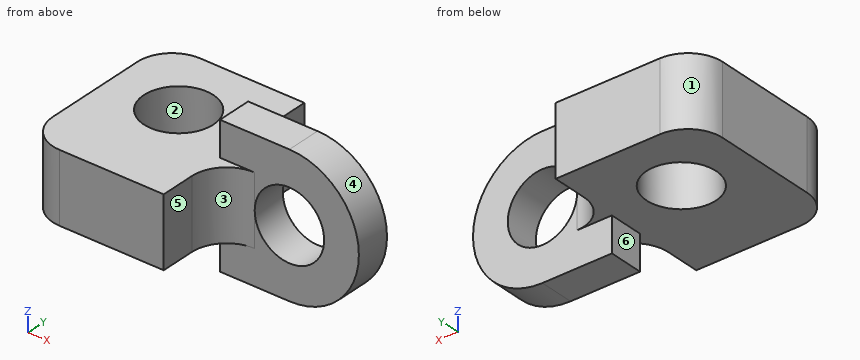
Autodesk Inventor part; units mm, degrees
ref_plane "工作平面1" through (0, 0, -10) normal (0, -1, 0) x (1, 0, 0)
ref_plane "YZ Plane" through (0, 0, 0) normal (1, 0, 0) x (0, 1, 0)
ref_plane "XZ Plane" through (0, 0, 0) normal (0, 1, 0) x (-1, 0, 0)
sketch "草圖1" plane through (0, 0, 0) normal (0, 0, 1) x (1, 0, 0)
  line L0 (-40, 25) -> (0, 25)
  line L1 (0, 25) -> (0, -25)
  line L2 (0, -25) -> (-40, -25)
  line L3 (-40, -25) -> (-40, 25)
  point P0 (0, 0)
  point P1 (0, 0)
  dimension "d0" = 50
  dimension "d1" = 40
extrude "擠出1" add sketch "草圖1" along normal mid plane 20
fillet "圓角1" radius 10 2 edges at (-40, 25, 0) (-40, -25, 0)
sketch "草圖2" plane through (0, 0, 10) normal (0, 0, 1) x (1, 0, 0)
  arc A0 (-40, -15) -> (-30, -25) centre (-30, -15) ccw
  line L0 (-40, -15) -> (-40, 15)
  arc A1 (-30, 25) -> (-40, 15) centre (-30, 15) ccw
  line L1 (-30, 25) -> (0, 25)
  line L2 (0, 25) -> (0, -25)
  line L3 (0, -25) -> (-30, -25)
  point P0 (0, 0)
  point P1 (-20, 5)
  dimension "d5" = 20
  dimension "d6" = 20
hole "孔1" at (-20, 5, 10) direction (0, 0, -1) diameter 20 end through all
ref_plane "工作平面1" through (0, 0, -10) normal (0, -1, 0) x (1, 0, 0)
sketch "草圖3" plane through (0, 0, -10) normal (0, -1, 0) x (1, 0, 0)
  line L0 (-11.3397, 0) -> (-11.3397, 20)
  line L1 (-11.3397, 20) -> (0, 20)
  line L2 (0, 20) -> (0, 0)
  line L3 (0, 0) -> (-11.3397, 0)
  line L4 (-28.6603, 20) -> (-28.6603, 0)
  line L5 (-28.6603, 0) -> (-40, 0)
  line L6 (-40, 0) -> (-40, 20)
  line L7 (-40, 20) -> (-28.6603, 20)
  circle A0 centre (20, 10) radius 20
  line L8 (20, -10) -> (0, -10)
  line L9 (0, -10) -> (0, 30)
  line L10 (0, 30) -> (20, 30)
  line L11 (20, 30) -> (20, -10)
  point P0 (0, 10)
  point P1 (0, 10)
  point P2 (20, 10)
  point P3 (0, 20)
  dimension "d15" = 40
  dimension "d14" = 20
extrude "擠出2" add sketch "草圖3" along normal mid plane 10 contours L2 A0 L8 L9 | L9 L10 A0 L2 | A0 L11 | A0 L11
fillet "圓角2" radius 10 2 edges at (0, 5, 0) (0, -5, 0)
sketch "草圖4" plane through (0, 5, -10) normal (0, 1, 0) x (1, 0, 0)
  arc A0 (20, -30) -> (20, 10) centre (20, -10) ccw
  point P0 (0, -10)
hole "孔2" at (20, 5, 0) direction (0, -1, 0) diameter 20 end through all
properties part number "22" material "鋼、碳鋼"
Read the model definition and answer for the solid it produces. Units are mm, in the model's axes. Face numbers are marked on the shaded views. A direction names the side the tool comes from. Give positions to 0.01 mm unless a question says otherwise; leave off trailing zeros. Loops run counter-clockwise (first coordinate to the right, second up) from the corner with the lowest first, then second, coordinate; pieces in that order, holes last. Notation, with made-up numbers: M 55.25,46 L 97.25,46 A17 ccw 97.25,60 Z; hole C -33,51.5 d9. An arc over 180 degrees is marked long. Write each question's results on one line, items separated by ' | '.
1. Section C-C on z = 1 is taken. Give the vertices of the cut face in (x, y), plus the area to 3 significant figures.
Values:
outline: M -40,-15 A10 ccw -30,-25 L 0,-25 L 0,-15 A10 cw 10,-5 L 10.05,-5 L 10.05,5 L 10,5 A10 cw 0,15 L 0,25 L -30,25 A10 ccw -40,15 Z; M 29.95,-5 L 39.97,-5 L 39.97,5 L 29.95,5 Z; hole C -20,5 d20 | area: 1,890 mm^2
2. Section D-D on y = 20 is taken. Give the vertices of the cut face in (x, z).
Values:
outline: M -38.66,-10 L 0,-10 L 0,10 L -38.66,10 Z
3. Given pin 1 (3 mm diameter, centred on y = 20, z = 0, fed in from +X); pin 2 (8 mm diameter, centred on y = 0, z = 15, fed in from -X); pin 3 (25 mm diameter, centred on x = -13, y = -8.5, fed in from -Z); pin 4 (18 mm diameter, centred on x = 20, z = 0, fed in from +Y), each flat-ended and moving along its own axis, determine where each tip first touches the part or whether it passes through.
Values:
pin 1: stops at x = 0 | pin 2: stops at x = 0 | pin 3: stops at z = -10 | pin 4: passes through
4. Straight lines are drawn through the part: line 1 (Y direction, x = -20, z = -2); line 2 (X direction, y = 0.5, z = 0); line 3 (X direction, y = 2, z = 0). For each, find the intervals that lie inside material, in ascending order. Write a range as [from, to].
Values:
line 1: y = [-25, -5], [15, 25] | line 2: x = [-40, -28.93], [-11.07, 10], [30, 40] | line 3: x = [-40, -29.54], [-10.46, 10], [30, 40]
5. The mould has two halves that part along Y. Classify the marked faces 1, 2 and 3: pulls with the +Y half, pulls with the -Y half, needs draft (parallel to the pull), parting line crosses it, or undercut.
Values:
face 1: pulls with the +Y half | face 2: undercut | face 3: pulls with the -Y half
6. Section B-B on x = 9 is taken. Give the vertices of the cut face in (y, z), plus the area to 3 significant figures.
Values:
outline: M -5.05,-10 L -5,-10 L -5,-20 L 5,-20 L 5,-10 L 5.05,-10 L 5.05,10 L 5,10 L 5,20 L -5,20 L -5,10 L -5.05,10 Z | area: 402 mm^2
7. Section A-A on z = -8 is taken. Give the vertices of the cut face in (x, y), plus the area to 3 significant figures.
Values:
outline: M -40,-15 A10 ccw -30,-25 L 0,-25 L 0,-15 A10 cw 10,-5 L 14,-5 L 14,5 L 10,5 A10 cw 0,15 L 0,25 L -30,25 A10 ccw -40,15 Z; M 26,-5 L 38.33,-5 L 38.33,5 L 26,5 Z; hole C -20,5 d20 | area: 1,950 mm^2
8. A tool of negligible diameter and unlimited length cuts with its end or side. For the marked faces 4, 5 and 6, from which of +Z, -Z, +X, -X, +Y, -Y can it reach the whole face along a straight path? Write none if from no direction.
Values:
face 4: +X, +Y, -Y | face 5: +Z, -Z, +X, -Y | face 6: -Z, -X, +Y, -Y
